Model file for the job. Use its own axes, mm. A direction names the side the tool comes from. Give positions to 0.01 mm unless a question says otherwise; leave off trailing zeros. Loops run counter-clockwise (first coordinate to the right, second up) from the corner with the lowest first, then second, coordinate; pieces in that order, holes last. Notation, with made-up numbers: (62.5, 46.25) - (117.5, 46.25) arc R13 ccw to (117.5, 70.25) - close; hole circle Ø4 at (2, 37.5). An arc over 180 degrees is marked (long way). Use a Markdown table: item, result.
from build123d import *

# Parameters (mm, degrees)
SKETCH1_R                = 3.75
BOSS_EXTRUDE1_DEPTH      = 2
BOSS_EXTRUDE2_DEPTH      = 65
BOSS_EXTRUDE2_DEPTH_BACK = 65
SKETCH4_R                = 12.5
SKETCH4_R_2              = 3.75
BOSS_EXTRUDE3_DEPTH      = 2
SKETCH5_R                = 12.5
CUT_EXTRUDE1_DEPTH       = 3
CUT_EXTRUDE1_DEPTH_BACK  = 29
BOSS_EXTRUDE4_DEPTH      = 26
SKETCH7_R                = 13
CUT_EXTRUDE2_DEPTH       = 66.0000001
CUT_EXTRUDE2_DEPTH_BACK  = 66.0000001
BOSS_EXTRUDE5_DEPTH      = 4
BOSS_EXTRUDE6_DEPTH      = 4


with BuildPart() as part:
    # Sketch1 → Boss-Extrude1 (new body)
    with BuildSketch(Plane.XY):
        with BuildLine():
            Line((-10.40198382, 6.931719311), (-65, -75))
            Line((-65, -75), (65, -75))
            Line((65, -75), (10.40198382, 6.931719311))
            ThreePointArc((10.40198382, 6.931719311), (0, 12.5), (-10.40198382, 6.931719311))
        make_face()
        Circle(SKETCH1_R, mode=Mode.SUBTRACT)
    extrude(amount=BOSS_EXTRUDE1_DEPTH)

    # Sketch2 → Boss-Extrude2 (add, two sides)
    with BuildSketch(Plane(origin=(0, 0, 0), x_dir=(0, 0, -1), z_dir=(1, 0, 0))) as boss_extrude2_sk:
        with BuildLine():
            Line((0, -75), (-2, -75))
            ThreePointArc((-2, -75), (13, -90), (28, -75))
            Line((28, -75), (26, -75))
            ThreePointArc((26, -75), (13, -88), (0, -75))
        make_face()
    extrude(amount=BOSS_EXTRUDE2_DEPTH)
    extrude(boss_extrude2_sk.sketch, amount=-BOSS_EXTRUDE2_DEPTH_BACK)

    # Sketch4 → Boss-Extrude3 (add)
    with BuildSketch(Plane(origin=(0, 0, -28), x_dir=(-1, 0, 0), z_dir=(0, 0, -1))):
        with BuildLine():
            ThreePointArc((12.5, 0), (-3.621132575, -11.964004299), (-10.40198382, 6.931719311))
            Line((-10.40198382, 6.931719311), (-65, -75))
            Line((-65, -75), (65, -75))
            Line((65, -75), (10.40198382, 6.931719311))
            ThreePointArc((10.40198382, 6.931719311), (11.964004299, 3.621132575), (12.5, 0))
        make_face()
        Circle(SKETCH4_R)
        Circle(SKETCH4_R_2, mode=Mode.SUBTRACT)
    extrude(amount=-BOSS_EXTRUDE3_DEPTH)

    # Sketch5 → Cut-Extrude1 (cut, two sides)
    with BuildSketch(Plane.XY) as cut_extrude1_sk:
        with Locations((0, -75)):
            Circle(SKETCH5_R)
    extrude(amount=CUT_EXTRUDE1_DEPTH, mode=Mode.SUBTRACT)
    extrude(cut_extrude1_sk.sketch, amount=-CUT_EXTRUDE1_DEPTH_BACK, mode=Mode.SUBTRACT)

    # Sketch6 → Boss-Extrude4 (add)
    with BuildSketch(Plane.XY):
        Polygon((15.021173144, 0), (13.021173144, 0), (63, -75), (65, -75), align=None)
        Polygon((-13.021173144, 0), (-15.021173144, 0), (-65, -75), (-63, -75), align=None)
    extrude(amount=-BOSS_EXTRUDE4_DEPTH)

    # Sketch7 → Cut-Extrude2 (cut, two sides)
    with BuildSketch(Plane(origin=(0, 0, 0), x_dir=(0, 0, -1), z_dir=(1, 0, 0))) as cut_extrude2_sk:
        with Locations((13, -75)):
            Circle(SKETCH7_R)
    extrude(amount=CUT_EXTRUDE2_DEPTH, mode=Mode.SUBTRACT)
    extrude(cut_extrude2_sk.sketch, amount=-CUT_EXTRUDE2_DEPTH_BACK, mode=Mode.SUBTRACT)

    # Sketch8 → Boss-Extrude5 (add)
    with BuildSketch(Plane(origin=(0, 0, -28), x_dir=(-1, 0, 0), z_dir=(0, 0, -1))):
        Polygon((8, 0), (4, 6.92820323), (-4, 6.92820323), (-8, 0), (-4, -6.92820323), (4, -6.92820323), align=None)
    extrude(amount=BOSS_EXTRUDE5_DEPTH)

    # Sketch9 → Boss-Extrude6 (add)
    with BuildSketch(Plane.XY.offset(2)):
        Polygon((8, 0), (4, 6.92820323), (-4, 6.92820323), (-8, 0), (-4, -6.92820323), (4, -6.92820323), align=None)
    extrude(amount=BOSS_EXTRUDE6_DEPTH)


solid = part.part
(1) Slice it at B-B, the plane x = 0. Write the cut outline in (y, z), plus the area to 3 significant figures.
Computed:
| item | result |
|---|---|
| outline | (-87.5, -21.29) - (-87.5, -16.57) arc R13 cw to (-87.5, -9.43) - (-87.5, -4.71) arc R15 ccw to start; (-62.5, -28) - (-6.93, -28) - (-6.93, -32) - (6.93, -32) - (6.93, -28) - (12.5, -28) - (12.5, -26) - (3.75, -26) - (3.75, -28) - (-3.75, -28) - (-3.75, -26) - (-62.5, -26) - close; (-62.5, 0) - (-3.75, 0) - (-3.75, 2) - (3.75, 2) - (3.75, 0) - (12.5, 0) - (12.5, 2) - (6.93, 2) - (6.93, 6) - (-6.93, 6) - (-6.93, 2) - (-62.5, 2) - close |
| area | 407 mm² |
(2) Slice it at A-A, the plane z = -12.5. Write the cut outline in (x, y).
Computed:
| item | result |
|---|---|
| outline | (-65, -89.99) - (65, -89.99) - (65, -87.99) - (-65, -87.99) - close; (-56.34, -62.01) - (-54.34, -62.01) - (-13.02, 0) - (-15.02, 0) - close; (13.02, 0) - (54.34, -62.01) - (56.34, -62.01) - (15.02, 0) - close |
(3) Slice it at D-D, the plane x = 51. Write the cut outline in (y, z), plus the area to 3 significant figures.
Computed:
| item | result |
|---|---|
| outline | (-75, -28) - (-53.99, -28) - (-53.99, 2) - (-75, 2) arc R15 ccw to start; hole (-75, -26) - (-56.99, -26) - (-56.99, 0) - (-75, 0) arc R13 ccw to start |
| area | 250 mm² |
(4) Slice it at C-C, the plane y = -12. Write the cut outline in (x, z).
Computed:
| item | result |
|---|---|
| outline | (-23.02, -28) - (23.02, -28) - (23.02, 2) - (-23.02, 2) - close; hole (-21.02, -26) - (21.02, -26) - (21.02, 0) - (-21.02, 0) - close |
(5) Drill centre lines: probe 1 along Z at (x, y) = (-27, -75); probe 2 along Y at (x, z) = (0, -26.75); probe 3 along Y at (x, z) = (53, -25). Where is each one in solid material? Low to high. Write a range as [from, to].
Computed:
| item | result |
|---|---|
| probe 1 | [-28, -26], [0, 2] |
| probe 2 | [-62.5, -3.75], [3.75, 12.5] |
| probe 3 | [-84, -80], [-59.99, -56.99] |
(6) Mould opens along X. For faces 1 (the cylindrical face through (-3.746, 0.165, 0.986)), 2 (the flat face through (-6.028, 3.416, -29.972)), 3 (the flat face through (0, -6.928, -30)) say: pulls with the +X half, pulls with the -X half, needs draft (parallel to the pull), parting line crosses it, or undercut.
Computed:
| item | result |
|---|---|
| face 1 | undercut |
| face 2 | pulls with the -X half |
| face 3 | needs draft |
(7) 3-axis set-ups, long thin cutter, end or side, ignore diameter. For faces 4 (the cylindrical face through (3.746, 0.165, -27.014)), 5 (the flat face through (0, 6.928, -30)), 6 (the cylindrical face through (-0.91, -87.69, -10.18)), 7 (the flat face through (0, -6.928, 4)): which of +Z, -Z, +X, -X, +Y, -Y reach the whole face in a straight line?
Computed:
| item | result |
|---|---|
| face 4 | none |
| face 5 | -Z, +X, -X, +Y |
| face 6 | +X, -X |
| face 7 | +Z, +X, -X, -Y |
(8) Pin check, flat tips, straight feed: P1, Ø10, axis at y = -58, z = -15.5, coming from the -X side; P2, Ø2, axis at x = -14, z = -9.5, coming from the +Y side; P3, Ø6, axis at x = 37.5, y = -66, coming from the +Z side. Stop position of each tip, or through.
Computed:
| item | result |
|---|---|
| P1 | x = -56.8 |
| P2 | y = 0 |
| P3 | z = 2 |
